Can you work these out from the drawing? Everything is in mm from the part's minimum corner. A direction names the side the tool comes from. Round coordinates to 2 decimals unless told otherwise and drop trailing zeros. Answer as CSV lines item,"result".
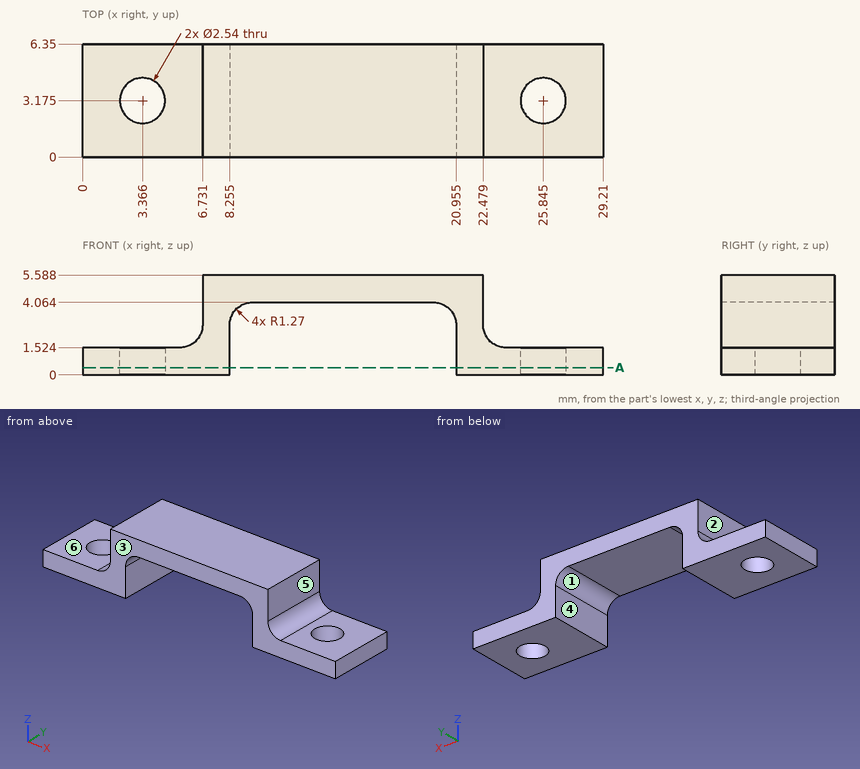
Item 1: I need wall thicknesses on L1, parallel to X at y = 4, z = 2.9; L2, parallel to X at y = 0.5, z = 1.3 (1 decimal); L3, parallel to Z at x = 25.75, y = 4.5 (1 decimal). Which ranges of each line are inside material? Lowest first, please.
Results found:
L1,"x = 6.73 to 8.26, 20.95 to 22.48"
L2,"x = 0 to 8.3, 21 to 29.2"
L3,"z = 0 to 1.5"
Item 2: Suppose I cut it at A-A, the plane z = 0.4. State how many separate pieces and enclosed holes the cut face has.
Results found:
separate pieces,"2"
enclosed holes,"2"
Item 3: Will these pins go through, and if not, where does the flat tip stop? pin 1 (0.8 mm diameter, centred on y = 2.5, z = 4, fed in from -X); pin 2 (1.5 mm diameter, centred on y = 4, z = 1.5, fed in from -X); pin 3 (0.8 mm diameter, centred on y = 4, z = 4.5, fed in from +X); pin 4 (1.6 mm diameter, centred on x = 26.5, y = 2, fed in from +Z).
Results found:
pin 1,"stops at x = 6.73"
pin 2,"stops at x = 0"
pin 3,"stops at x = 22.48"
pin 4,"stops at z = 1.52"
Item 4: For the marked faces 4, 5 and 6, which set-ups out of +Z, -Z, +X, -X, +Y, -Y let a thin tool reach every point of the face, with its end or its side?
Results found:
face 4,"-Z, +Y, -Y"
face 5,"+Z, +X, +Y, -Y"
face 6,"+Z, -X, +Y, -Y"
Item 5: If we mould it in two halves opening along X, with no side actions, what happens to the marked faces 1, 2 and 3? For each: pulls with the +X half, pulls with the -X half, needs draft (parallel to the pull), parting line crosses it, or undercut.
Results found:
face 1,"undercut"
face 2,"pulls with the -X half"
face 3,"needs draft"
